```python
from build123d import *

# Parameters (mm, degrees)
SKETCH3_W           = 50
SKETCH3_H           = 90
BOSS_EXTRUDE2_DEPTH = 1.6
CUT_EXTRUDE1_REACH  = 3.6
SKETCH4_R           = 1.854
SKETCH5_W           = 8
SKETCH5_H           = 5
BOSS_EXTRUDE3_DEPTH = 3


with BuildPart() as part:
    # Sketch3 → Boss-Extrude2 (new body)
    with BuildSketch(Plane(origin=(0, 0, 0), x_dir=(1, 0, 0), z_dir=(0, 1, 0))):
        with Locations((25, -45)):
            Rectangle(SKETCH3_W, SKETCH3_H)
    extrude(amount=BOSS_EXTRUDE2_DEPTH)

    # Sketch4 → Cut-Extrude1 (cut, up to next)
    with BuildSketch(Plane(origin=(0, 1.6, 0), x_dir=(1, 0, 0), z_dir=(0, 1, 0)), mode=Mode.PRIVATE) as cut_extrude1_sk1:
        with Locations((3, -3.002549058)):
            Circle(SKETCH4_R)
    cut_extrude1_tool1 = extrude(cut_extrude1_sk1.sketch, amount=-CUT_EXTRUDE1_REACH, mode=Mode.PRIVATE) & part.part
    add(cut_extrude1_tool1.solids().sort_by_distance((3, 1.6, 3.002549))[0], mode=Mode.SUBTRACT)
    # Sketch4 → Cut-Extrude1 (cut, up to next)
    with BuildSketch(Plane(origin=(0, 1.6, 0), x_dir=(1, 0, 0), z_dir=(0, 1, 0)), mode=Mode.PRIVATE) as cut_extrude1_sk2:
        with Locations((47, -3.002549058)):
            Circle(SKETCH4_R)
    cut_extrude1_tool2 = extrude(cut_extrude1_sk2.sketch, amount=-CUT_EXTRUDE1_REACH, mode=Mode.PRIVATE) & part.part
    add(cut_extrude1_tool2.solids().sort_by_distance((47, 1.6, 3.002549))[0], mode=Mode.SUBTRACT)
    # Sketch4 → Cut-Extrude1 (cut, up to next)
    with BuildSketch(Plane(origin=(0, 1.6, 0), x_dir=(1, 0, 0), z_dir=(0, 1, 0)), mode=Mode.PRIVATE) as cut_extrude1_sk3:
        with Locations((47, -87.002549058)):
            Circle(SKETCH4_R)
    cut_extrude1_tool3 = extrude(cut_extrude1_sk3.sketch, amount=-CUT_EXTRUDE1_REACH, mode=Mode.PRIVATE) & part.part
    add(cut_extrude1_tool3.solids().sort_by_distance((47, 1.6, 87.002549))[0], mode=Mode.SUBTRACT)
    # Sketch4 → Cut-Extrude1 (cut, up to next)
    with BuildSketch(Plane(origin=(0, 1.6, 0), x_dir=(1, 0, 0), z_dir=(0, 1, 0)), mode=Mode.PRIVATE) as cut_extrude1_sk4:
        with Locations((3, -87.002549058)):
            Circle(SKETCH4_R)
    cut_extrude1_tool4 = extrude(cut_extrude1_sk4.sketch, amount=-CUT_EXTRUDE1_REACH, mode=Mode.PRIVATE) & part.part
    add(cut_extrude1_tool4.solids().sort_by_distance((3, 1.6, 87.002549))[0], mode=Mode.SUBTRACT)

    # Sketch5 → Boss-Extrude3 (add)
    with BuildSketch(Plane(origin=(0, 1.6, 0), x_dir=(1, 0, 0), z_dir=(0, 1, 0))):
        with Locations((9.8, -2.5)):
            Rectangle(SKETCH5_W, SKETCH5_H)
    extrude(amount=BOSS_EXTRUDE3_DEPTH)


solid = part.part
```
Can you work these out from the model? Positions are in its coordinate system, mm. A direction names the side the tool comes from. Coordinates: 2 decimals unless noted, no trailing zeros. Write each loop counter-clockwise with the first axis right and the second up, starting at its lowest first coordinate (ties: lowest second). Pieces come first, ordered by that corner, then holes. Notation, with made-up numbers: M -12,13 L 18,13 A26 cw 18,32 Z; hole C 74,59.5 d5. An arc over 180 degrees is marked long. Write item = value, one per line. Start each with the question number.
Q1. On a 3-axis mill with a long thin cutter (end or side, diameter ignored), from which of +Z, -Z, +X, -X, +Y, -Y can I reach the whole of each face in a straight line? I mean faces 4 (the face through (46.598, 0.811, 88.812)), 5 (the face through (13.8, 3, 3)), 6 (the face through (5.8, 3, 3)). Say none if no direction works.
Q2. Thinking about a two-plate mould opening in Z: for faces 1 (the face through (48.77, 0.81, 2.45)), 2 (the face through (50, 1, 46)), 3 (the face through (10, 3, 5)), which applies, released by +Z, released by -Z, zero draft, split by the parting line, or undercut?
Q3. If we section it at C-C, the plane x = 10: Write out the boundary of the cut face in (y, z), then the cut area to 3 significant figures.
Q4. I'm going to push flat-ended pins straight in: pin 1 (2 mm diameter, centred on y = 0.5, z = 52.5, fed in from -X); pin 2 (6 mm diameter, centred on x = 47, z = 87, fed in from +Y); pin 3 (3.5 mm diameter, centred on x = 3, z = 87, fed in from +Y); pin 4 (0.9 mm diameter, centred on y = 3, z = 1.5, fed in from -X). Where does each tip first touch, or does it pass through?
Q5. If we section it at A-A, the plane x = 47: Write out the boundary of the cut face in (y, z), then the cut area to 3 significant figures.
Q6. If we section it at B-B, the plane z = 61.5: Write out the boundary of the cut face in (x, y).
Q7. If I drill on L1, parallel to Z at x = 47, y = 1.2; L2, parallel to Y at x = 37.5, z = 66; L3, parallel to X at y = 1.65, z = 4, over which ranges is the centre line in solid material (lowest first)? Write a range as [from, to].
Q8. If we section it at D-D, the plane y = 3.7: Write out the boundary of the cut face in (x, z).
Check sheet entries:
q1.face_4 = +Y, -Y
q1.face_5 = +Z, -Z, +X, +Y
q1.face_6 = +Z, -Z, -X, +Y
q2.face_1 = undercut
q2.face_2 = zero draft
q2.face_3 = released by +Z
q3.outline = M 0,0 L 4.6,0 L 4.6,5 L 1.6,5 L 1.6,90 L 0,90 Z
q3.area = 159 mm²
q4.pin_1 = 0
q4.pin_2 = 1.6
q4.pin_3 = through
q4.pin_4 = 5.8
q5.outline = M 0,0 L 1.6,0 L 1.6,1.15 L 0,1.15 Z; M 0,4.86 L 1.6,4.86 L 1.6,85.15 L 0,85.15 Z; M 0,88.86 L 1.6,88.86 L 1.6,90 L 0,90 Z
q5.area = 132 mm²
q6.outline = M 0,0 L 50,0 L 50,1.6 L 0,1.6 Z
q7.L1 = [0, 1.15], [4.86, 85.15], [88.86, 90]
q7.L2 = [0, 1.6]
q7.L3 = [5.8, 13.8]
q8.outline = M 5.8,0 L 13.8,0 L 13.8,5 L 5.8,5 Z
